Drawing for the job (mm, zero at the part's lowest x, y, z). Round coordinates to 2 decimals unless told otherwise and drop trailing zeros. Loops run counter-clockwise (first coordinate to the right, second up) from the corner with the lowest first, then second, coordinate; pieces in that order, holes last. Notation, with made-up numbers: M 76,-22.5 L 107,-22.5 A13 ccw 107,-6.5 Z; hole C 53,-33 d10. An arc over 180 degrees is marked long. Write each question's results on one line, items separated by ' | '.
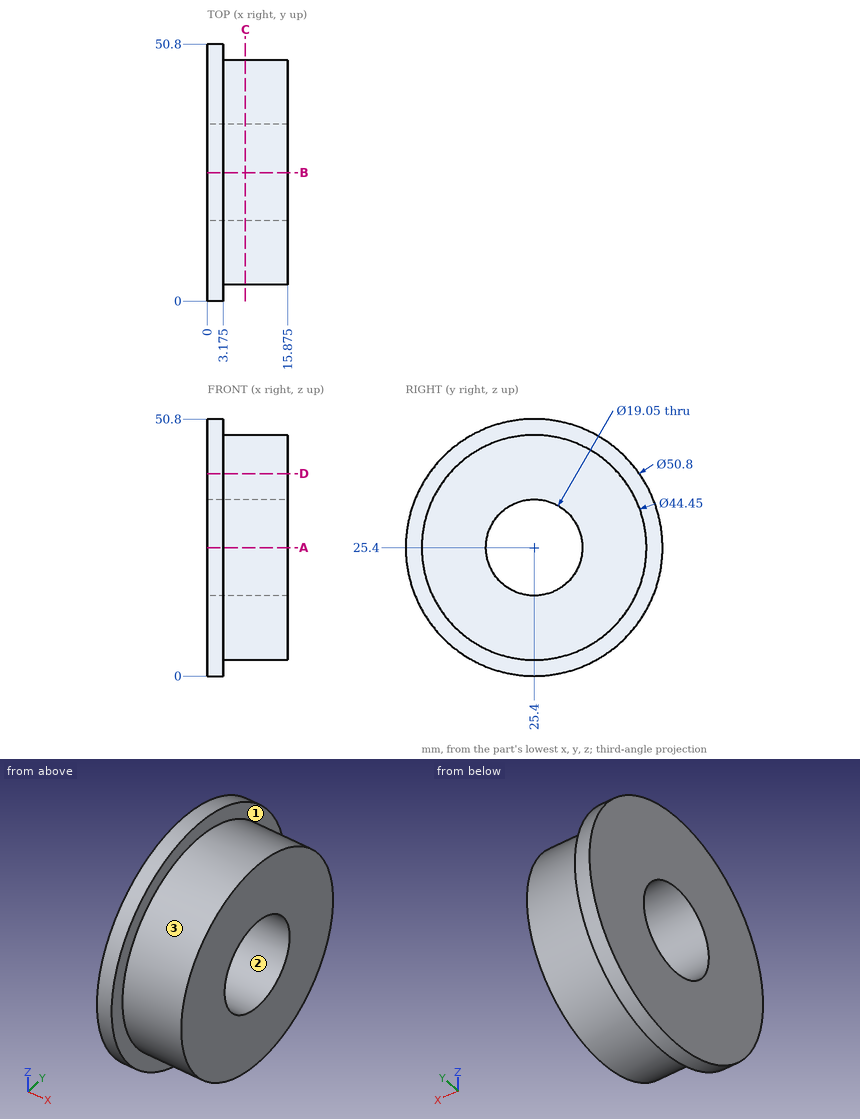
Item 1: Band-saw the part on C-C on x = 7.5. Give the cut face in (y, z) (3 decimals).
Filled sheet:
outline: C 25.4,25.4 d44.45; hole C 25.4,25.4 d19.05
Item 2: Drop flat-ended pins along their axis: P1, Ø5, axis at x = 2.5, z = 36, coming from the -Y side; P2, Ø1.5, axis at x = 7.5, y = 33, coming from the +Z side; P3, Ø3, axis at x = 10.5, z = 10, coming from the -Y side; P4, Ø1, axis at y = 44.5, z = 30.5, coming from the -X side. Give the stop position or say it passes through.
Filled sheet:
P1: y = 1.33 | P2: z = 46.54 | P3: y = 8.06 | P4: x = 0
Item 3: Wall check: L1, parallel to Y at x = 11.75, z = 25.4 (3 decimals); L2, parallel to Z at x = 1.75, y = 22; L3, parallel to Z at x = 12.5, y = 22. Give the ranges that are in metal, low to high.
Filled sheet:
L1: 3.175 to 15.875, 34.925 to 47.625 | L2: 0.23 to 16.5, 34.3 to 50.57 | L3: 3.44 to 16.5, 34.3 to 47.36
Item 4: Band-saw the part on D-D on z = 40. Give the cut face in (x, y) (3 decimals), and give its area (3 significant figures).
Filled sheet:
outline: M 0,4.615 L 3.175,4.615 L 3.175,8.643 L 15.875,8.643 L 15.875,42.157 L 3.175,42.157 L 3.175,46.185 L 0,46.185 Z | area: 558 mm^2
Item 5: Two-plate mould, pull along Y, no slides. Class the marked faces 1, 2 and 3: +Y half, -Y half, draft (parallel to the pull), parting line (faces both ways), or undercut.
Filled sheet:
face 1: draft | face 2: undercut | face 3: parting line
Item 6: Band-saw the part on A-A on z = 25.4. Give the cut face in (x, y) (3 decimals).
Filled sheet:
outline: M 0,0 L 3.175,0 L 3.175,3.175 L 15.875,3.175 L 15.875,15.875 L 0,15.875 Z; M 0,34.925 L 15.875,34.925 L 15.875,47.625 L 3.175,47.625 L 3.175,50.8 L 0,50.8 Z
